Source: three-view drawing plus pictorial views. Frame: mm from the lowest corner of the part. A direction names the side the tool comes from. Give positions to 0.01 mm unless a question says otherwise; leave off trailing zeros. Order: outer loops, then holes, each group sorted by start corner. A loop starts at its lowest first (then second) coordinate and runs counter-clockwise, first axis right, second up. Notation, with made-up numbers: (-2, 26.5) - (28, 26.5) arc R17 ccw to (28, 43.5) - close; hole circle Ø8 at (65, 77.25). An arc over 180 degrees is marked (long way). Answer in a Markdown table with one row per item. Add a question column.
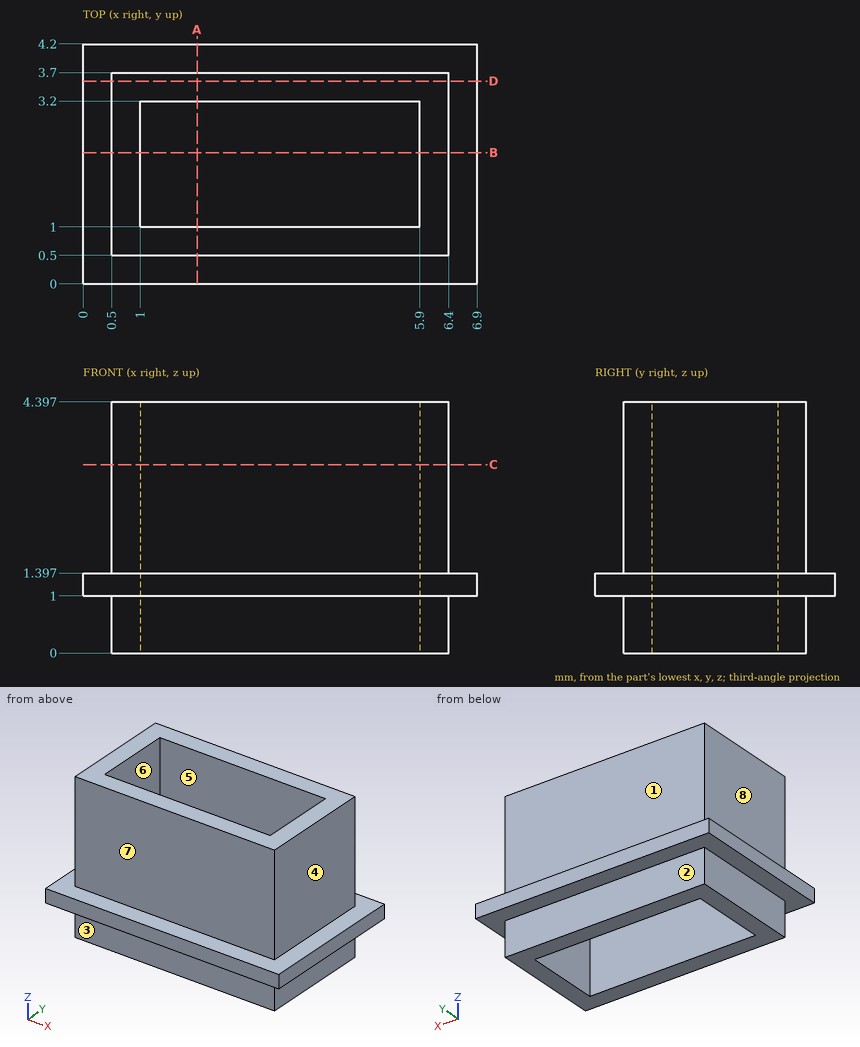
Q1. Pull-direction query (X, two-part tool) for the marked faces 6, 7 and 8; classes: +X half, -X half, draft (parallel to the pull), parting line (faces both ways), or undercut.
Q2. Line query: probe 1 along X at (y, z) = (1.1, 1.2); probe 2 along X at (y, z) = (2.55, 2.5); probe 3 along Y at (x, z) = (4, 2.85). Output: solid intervals per line, ascending.
Q3. Section C-C, the plane z = 3.3. Return loops of the section in (x, y).
Q4. Contact query for flat-ended pins moving along their axis: P1, Ø0.9, axis at y = 2, z = 2.5, coming from the -X side; P2, Ø0.9, axis at y = 2.5, z = 2.5, coming from the +X side; P3, Ø1.3, axis at x = 4, y = 2.5, coming from the -Z side; P4, Ø0.7, axis at y = 2, z = 1.5, coming from the +X side. Output: stop coordinate, or through.
Q5. Section D-D, the plane y = 3.55. Return loops of the section in (x, z).
Q6. Access query for the marked faces 1, 2, 3, 4 and 5. Directions: +Z, -Z, +X, -X, +Y, -Y. A direction counts if a zero-diameter tool reaches every point of the face in a straight line with its end or side. Return the directions, or none.
Q7. Section B-B, the plane y = 2.3. Return loops of the section in (x, z).
Q8. Section A-A, the plane x = 2. Return loops of the section in (y, z).
Computed:
| question | item | result |
|---|---|---|
| 1 | face 6 | undercut |
| 1 | face 7 | draft |
| 1 | face 8 | -X half |
| 2 | probe 1 | x = 0 to 1, 5.9 to 6.9 |
| 2 | probe 2 | x = 0.5 to 1, 5.9 to 6.4 |
| 2 | probe 3 | y = 0.5 to 1, 3.2 to 3.7 |
| 3 | outline | (0.5, 0.5) - (6.4, 0.5) - (6.4, 3.7) - (0.5, 3.7) - close; hole (1, 1) - (5.9, 1) - (5.9, 3.2) - (1, 3.2) - close |
| 4 | P1 | stops at x = 0.5 |
| 4 | P2 | stops at x = 6.4 |
| 4 | P3 | passes through |
| 4 | P4 | stops at x = 6.9 |
| 5 | outline | (0, 1) - (0.5, 1) - (0.5, 0) - (6.4, 0) - (6.4, 1) - (6.9, 1) - (6.9, 1.4) - (6.4, 1.4) - (6.4, 4.4) - (0.5, 4.4) - (0.5, 1.4) - (0, 1.4) - close |
| 6 | face 1 | +Z, +X, -X, +Y |
| 6 | face 2 | -Z, +X, -X, +Y |
| 6 | face 3 | -Z, +X, -X, -Y |
| 6 | face 4 | +Z, +X, +Y, -Y |
| 6 | face 5 | +Z, -Z |
| 7 | outline | (0, 1) - (0.5, 1) - (0.5, 0) - (1, 0) - (1, 4.4) - (0.5, 4.4) - (0.5, 1.4) - (0, 1.4) - close; (5.9, 0) - (6.4, 0) - (6.4, 1) - (6.9, 1) - (6.9, 1.4) - (6.4, 1.4) - (6.4, 4.4) - (5.9, 4.4) - close |
| 8 | outline | (0, 1) - (0.5, 1) - (0.5, 0) - (1, 0) - (1, 4.4) - (0.5, 4.4) - (0.5, 1.4) - (0, 1.4) - close; (3.2, 0) - (3.7, 0) - (3.7, 1) - (4.2, 1) - (4.2, 1.4) - (3.7, 1.4) - (3.7, 4.4) - (3.2, 4.4) - close |
